Part model, mm, in its own coordinate system. A direction names the side the tool comes from. Give positions to 0.01 mm unless a question says otherwise; leave off trailing zeros. Write each loop counter-clockwise with the first axis right and the second up, starting at its lowest first coordinate (ties: lowest second). Pieces come first, ordered by that corner, then holes.
```python
from build123d import *

# Parameters (mm, degrees)
SKETCH1_W                    = 80
SKETCH1_H                    = 80
BOSS_EXTRUDE1_DEPTH          = 52
CHAMFER1_SIZE                = 15
CUT_EXTRUDE_THIN2_DEPTH      = 77.837490849
CUT_EXTRUDE_THIN2_DEPTH_BACK = 77.837490849
SKETCH3_R                    = 10.96
CUT_EXTRUDE2_DEPTH           = 16


with BuildPart() as part:
    # Sketch1 → Boss-Extrude1 (new body)
    with BuildSketch(Plane.XY):
        Rectangle(SKETCH1_W, SKETCH1_H)
    extrude(amount=BOSS_EXTRUDE1_DEPTH)

    # Chamfer1
    chamfer1_edges = [part.edges().sort_by_distance(p)[0] for p in [
        (40, -40, 26),
        (-40, -40, 26),
        (-40, 40, 26),
        (40, 40, 26),
    ]]
    chamfer(chamfer1_edges, length=CHAMFER1_SIZE)

    # Sketch2 → Cut-Extrude-Thin2 (cut, two sides: drawn at the far end of the back side and taken through both)
    with BuildSketch(Plane(origin=(0, 0, 0), x_dir=(-1, 0, 0), z_dir=(0, 0, -1)).offset(-CUT_EXTRUDE_THIN2_DEPTH_BACK)):
        Polygon((44.0879895, 11), (15.722057871, 11), (22.061953445, 16.76959481), (-12.810565673, 16.76959481), (-12.810565673, 17.76959481), (24.646552449, 17.76959481), (18.306656875, 12), (44.0879895, 12), align=None)
        Polygon((-43.151938768, -11), (-15.722057871, -11), (-22.061953445, -16.76959481), (12.810565673, -16.76959481), (12.810565673, -17.76959481), (-24.646552449, -17.76959481), (-18.306656875, -12), (-43.151938768, -12), align=None)
    extrude(amount=CUT_EXTRUDE_THIN2_DEPTH + CUT_EXTRUDE_THIN2_DEPTH_BACK, mode=Mode.SUBTRACT)

    # Sketch3 → Cut-Extrude2 (cut)
    with BuildSketch(Plane(origin=(0, 40, 0), x_dir=(1, 0, 0), z_dir=(0, 1, 0))):
        with Locations(Location((0, -26, 0), (0, 0, 270))):
            Circle(SKETCH3_R)
    cut_extrude2 = extrude(amount=-CUT_EXTRUDE2_DEPTH, mode=Mode.SUBTRACT)

    # Mirror1: Cut-Extrude2 across plane
    add(cut_extrude2.mirror(Plane.ZX), mode=Mode.SUBTRACT)


solid = part.part
```
1) 3-axis set-ups, long thin cutter, end or side, ignore diameter. For faces 1 (the face through (3.292, -32.112, 36.454)), 2 (the face through (-5, 16.77, 26)), 3 (the face through (-28, 11, 26)), 4 (the face through (29, -12, 26)), 5 (the face through (0, 24, 26)): which of +Z, -Z, +X, -X, +Y, -Y reach the whole face in a straight line?
Answers follow:
face 1: -Y
face 2: +Z, -Z
face 3: +Z, -Z, -X
face 4: +Z, -Z, +X
face 5: +Y
2) Wall check: L1, parallel to Y at x = 4, z = 21; L2, parallel to Y at x = 6.5, z = 9.5; L3, parallel to Y at x = 18.5, z = 9. Give the ranges that are in metal, low to high.
Answers follow:
L1: y = -24 to -17.77, -16.77 to 16.77, 17.77 to 24
L2: y = -40 to -17.77, -16.77 to 16.77, 17.77 to 40
L3: y = -40 to -17.77, -16.77 to -13.53, -12.18 to -12, -11 to 40
3) Saw through at C-C, the plane x = -20.5. Write the cut outline in (y, z), then the cut area to 3 significant figures.
Answers follow:
outline: (-40, 0) - (11, 0) - (11, 52) - (-40, 52) - close; (12, 0) - (14, 0) - (14, 52) - (12, 52) - close; (15.35, 0) - (16.77, 0) - (16.77, 52) - (15.35, 52) - close; (17.77, 0) - (40, 0) - (40, 52) - (17.77, 52) - close
area: 3,990 mm2
4) Saw through at A-A, the plane x = 0. Write the cut outline in (y, z).
Answers follow:
outline: (-40, 0) - (-17.77, 0) - (-17.77, 52) - (-40, 52) - (-40, 36.96) - (-24, 36.96) - (-24, 15.04) - (-40, 15.04) - close; (-16.77, 0) - (16.77, 0) - (16.77, 52) - (-16.77, 52) - close; (17.77, 0) - (40, 0) - (40, 15.04) - (24, 15.04) - (24, 36.96) - (40, 36.96) - (40, 52) - (17.77, 52) - close
5) Pin check, flat tips, straight feed: pin 1 Ø6.5 at (x, z) = (-31, 17.5) entering from -Y; pin 2 Ø17.5 at (x, z) = (0, 26) entering from +Y; pin 3 Ø1 at (y, z) = (-29, 14) entering from -X. Stop position of each tip, or through.
Answers follow:
pin 1: stops at y = -37.25
pin 2: stops at y = 24
pin 3: stops at x = -36.5
6) Saw through at D-D, the plane y = -27.5. Write the cut outline in (x, z), then the cut area to 3 significant figures.
Answers follow:
outline: (-37.5, 0) - (37.5, 0) - (37.5, 52) - (-37.5, 52) - close; hole circle Ø21.92 at (0, 26)
area: 3,520 mm2
7) Two-plate mould, pull along X, no slides. Class faces 6 (the face through (40, 7, 26)), 7 (the face through (-21.521, 14.925, 26.364)), 8 (the face through (-40, 18, 26)): +X half, -X half, draft (parallel to the pull), parting line (faces both ways), or undercut.
Answers follow:
face 6: +X half
face 7: undercut
face 8: -X half
